Geometry: see drawing. Coordinates: mm, zero at the bounding-box minimum. A direction names the side the tool comes from. Coordinates: 2 decimals unless noted, no trailing zeros. Write each loop counter-clockwise with the first axis right and the second up, starting at its lowest first coordinate (ties: lowest second). Pieces come first, ordered by that corner, then holes. Notation, with made-up numbers: (67.5, 62.25) - (125.5, 62.25) arc R24 cw to (125.5, 100.25) - close; hole circle Ø10 at (19, -1). An arc over 180 degrees is marked (long way). Use CSV: the item, a comma, the result in double quotes.
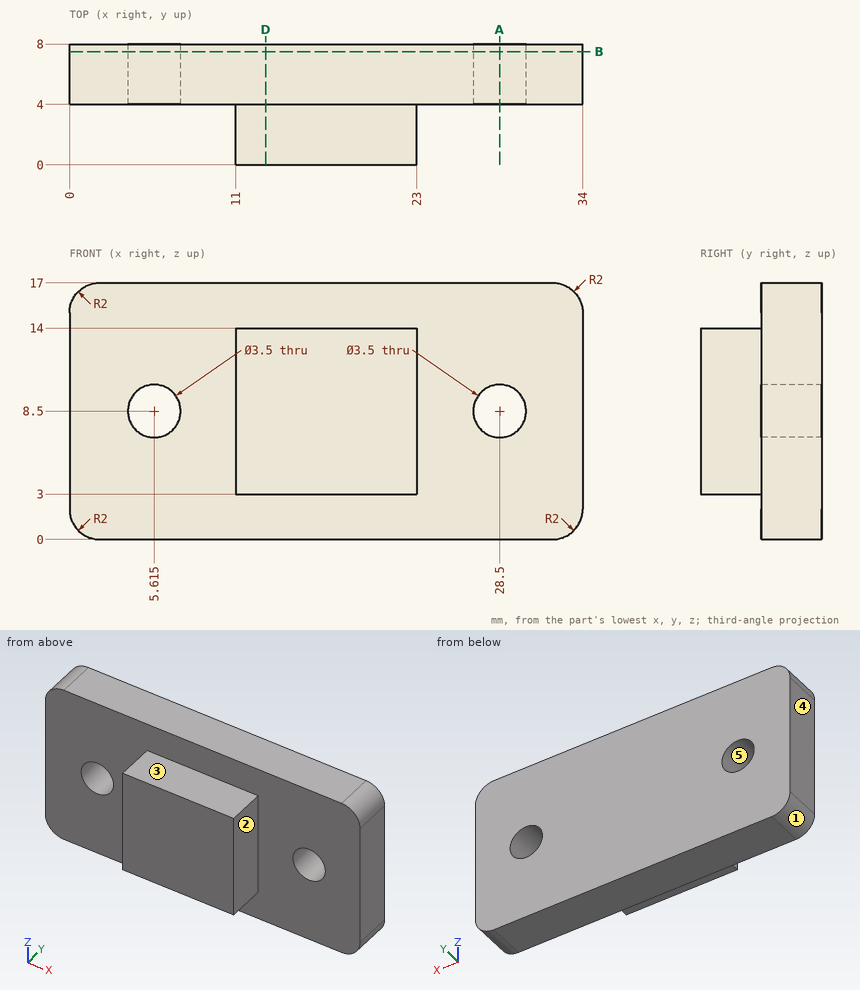
(1) Cut plane A-A on x = 28.5. Return loops of the section in (y, z), and give its area (3 significant figures).
Check values:
outline,"(4, 0) - (8, 0) - (8, 6.75) - (4, 6.75) - close; (4, 10.25) - (8, 10.25) - (8, 17) - (4, 17) - close"
area,"54.0 mm^2"
(2) Draft query along Z for the marked faces 3, 4 and 5. Return one class per face: pulls with the +Z half, pulls with the -Z half, needs draft (parallel to the pull), parting line crosses it, or undercut.
Check values:
face 3,"pulls with the +Z half"
face 4,"needs draft"
face 5,"undercut"
(3) Cut plane B-B on y = 7.5. State how many separate pieces and enclosed holes the cut face has, and give its area (3 significant figures).
Check values:
separate pieces,"1"
enclosed holes,"2"
area,"555 mm^2"
(4) Ray query, probe 1 along Z at (x, y) = (28.5, 5.65); probe 2 along X at (y, z) = (7, 10) (1 decimal); probe 3 along Z at (x, y) = (22.5, 1.5). Return the intervals inside material, ascending. Write a range as from..to.
Check values:
probe 1,"0..6.75, 10.25..17"
probe 2,"0..4.7, 6.5..27.6, 29.4..34"
probe 3,"3..14"
(5) Pin query (flat end, axial travel): pin 1 Ø2 at (y, z) = (2, 9.5) entering from -X; pin 2 Ø5 at (x, z) = (8.5, 2) entering from -Y; pin 3 Ø2 at (x, y) = (18.5, 2) entering from +Z. Return the tip coordinate at first contact, or that it passes through.
Check values:
pin 1,"x = 11"
pin 2,"y = 4"
pin 3,"z = 14"
(6) Reachability of the marked faces 1 and 2 from +Z, -Z, +X, -X, +Y, -Y: full face, straight path, thin tool, end or side. Return the list, or none.
Check values:
face 1,"-Z, -X, +Y, -Y"
face 2,"+Z, -Z, +X, -Y"
(7) Cut plane D-D on x = 13. Return loops of the section in (y, z).
Check values:
outline,"(0, 3) - (4, 3) - (4, 0) - (8, 0) - (8, 17) - (4, 17) - (4, 14) - (0, 14) - close"
